Geometry: final body of the model. Coordinates: model frame, mm. A direction names the side the tool comes from. Coordinates: 2 decimals unless noted, no trailing zeros. Write each loop counter-clockwise with the first axis right and the second up, starting at its lowest first coordinate (ties: lowest second). Pieces come first, ordered by that corner, then holes. Notation, with made-up numbers: (12.5, 83.5) - (30.5, 83.5) arc R28 ccw to (30.5, 105.5) - close; hole circle Ø4 at (52.5, 25). An arc over 180 degrees is marked (long way). Answer as a JSON object with one key per item and string values. Group by question number.
Item 1: Section C-C on y = 26. Return loops of the section in (x, z).
Item 2: Set-up query: faces 4 (the flat face through (58.6, 0, 53)), 5 (the flat face through (-1, 1, 1)), 6 (the flat face through (60, -2.5, 50)). Return all of +Z, -Z, +X, -X, +Y, -Y with unobstructed straight access to the full face (end or side cutting, diameter ignored); none if empty.
Item 3: Mould query, pull axis Y, two halves, no side actions, for faces 1 (the flat face through (37, -8, 120)), 2 (the cylindrical face through (-37.18, 4.88, 61.33)), 3 (the flat face through (60, 2.5, 50)). Classes: pulls with the +Y half, pulls with the -Y half, needs draft (parallel to the pull), parting line crosses it, or undercut.
Item 4: Section A-A on z = 46. Return loops of the section in (x, y), and give its area (3 significant figures).
Item 5: Line query: line 1 along X through (y, z) = (0, 43); line 2 along Y through (x, z) = (0, 94); line 3 along X through (y, z) = (-6, 72). Output: solid intervals per line, ascending. Write a range as from..to.
Item 6: First-contact query: pin 1 Ø12 at (x, z) = (-19.5, 53) entering from -Y; pin 2 Ø1 at (x, z) = (-3, 55.5) entering from -Y; pin 3 Ø10.5 at (x, z) = (47.5, 32.5) entering from -Y; pin 4 Ø1.5 at (x, y) = (-2.5, -8.5) entering from -Z. Flat tips, straight axial feed; report the tip coordinate or a pass-through.
Item 7: Section D-D on x = 52.5. Return loops of the section in (y, z).
Item 8: Section B-B on x = 0. Return loops of the section in (y, z).
```python
from build123d import *

# Parameters (mm, degrees)
F0_W     = 38.5
F0_H     = 120
F2_T     = -1
F4_DEPTH = 2.5


with BuildPart() as f1:
    # F0 (on Right) → F1 (revolve)
    with BuildSketch(Plane.YZ):
        with Locations((-19.25, 60)):
            Rectangle(F0_W, F0_H)
    revolve(axis=Axis((0, 0, 60), (0, 0, -1)))

    # F2
    f2_openings = [f1.faces().sort_by_distance(p)[0] for p in [
        (0, 0, 120),
    ]]
    offset(amount=F2_T, openings=f2_openings)

    # F3 (on Front) → F4 (join, symmetric)
    with BuildSketch(Plane.XZ):
        Polygon((73.600475, 69.767932), (38.349035, 88.511455), (38.184893, 79.107806), (58.600475, 68.252649), (58.600475, 38.252649), (37.887409, 25.309689), (37.887409, 10.546948), (73.600475, 32.862948), align=None)
    extrude(amount=F4_DEPTH, both=True)


solid = f1.part
```
Checks:
{
 "1": {"outline": "(-28.39, 0) - (28.39, 0) - (28.39, 120) - (27.02, 120) - (27.02, 1) - (-27.02, 1) - (-27.02, 120) - (-28.39, 120) - close"},
 "2": {"face 4": "+Y, -Y", "face 5": "+Z", "face 6": "+Z, -Z, +X, -Y"},
 "3": {"face 1": "needs draft", "face 2": "undercut", "face 3": "pulls with the +Y half"},
 "4": {"outline": "circle Ø77 at (0, 0); (58.6, -2.5) - (73.6, -2.5) - (73.6, 2.5) - (58.6, 2.5) - close; hole circle Ø75 at (0, 0)", "area": "314 mm^2"},
 "5": {"line 1": "-38.5..-37.5, 37.5..38.5, 58.6..73.6", "line 2": "-38.5..-37.5, 37.5..38.5", "line 3": "-38.03..-37.02, 37.02..38.03"},
 "6": {"pin 1": "y = -36.06", "pin 2": "y = -38.42", "pin 3": "y = -2.5", "pin 4": "z = 0"},
 "7": {"outline": "(-2.5, 19.68) - (2.5, 19.68) - (2.5, 34.44) - (-2.5, 34.44) - close; (-2.5, 71.5) - (2.5, 71.5) - (2.5, 80.99) - (-2.5, 80.99) - close"},
 "8": {"outline": "(-38.5, 0) - (38.5, 0) - (38.5, 120) - (37.5, 120) - (37.5, 1) - (-37.5, 1) - (-37.5, 120) - (-38.5, 120) - close"}
}
